```python
from build123d import *

# Parameters (mm, degrees)
CYLINDER023_R       = 1.8
CYLINDER023_DEPTH   = 20
ARRAY001003_X_COUNT = 2
ARRAY001003_X_PITCH = 31
ARRAY001003_Y_COUNT = 2
ARRAY001003_Y_PITCH = 31
CYLINDER020_R       = 13
CYLINDER020_DEPTH   = 30
CYLINDER024_R       = 30
CYLINDER024_DEPTH   = 30
CYLINDER039_R       = 1.45
CYLINDER039_DEPTH   = 40
ARRAY001020_X_COUNT = 2
ARRAY001020_X_PITCH = 20
ARRAY001021_X_COUNT = 2
ARRAY001021_X_PITCH = 90
CYLINDER041_R       = 1
CYLINDER041_DEPTH   = 10
ARRAY001023_Y_COUNT = 2
ARRAY001023_Y_PITCH = 92
CYLINDER022_R       = 4.1
CYLINDER022_DEPTH   = 24
ARRAY001002_X_COUNT = 2
ARRAY001002_X_PITCH = 90
ARRAY001002_Y_COUNT = 2
ARRAY001002_Y_PITCH = 50
CYLINDER025_R       = 7
CYLINDER025_DEPTH   = 25
ARRAY001004_X_COUNT = 2
ARRAY001004_X_PITCH = 90
ARRAY001004_Y_COUNT = 2
ARRAY001004_Y_PITCH = 50
BOX020_W            = 30
BOX020_H            = 100
BOX020_DEPTH        = 10
BOX002_W            = 120
BOX002_H            = 84
BOX002_DEPTH        = 10


with BuildPart() as motor_attachment_hole_array:
    # Cylinder023 → Cylinder023 (new body)
    with BuildSketch(Plane(origin=(84.5, 24.5, 0), x_dir=(1, 0, 0), z_dir=(0, 0, 1))):
        Circle(CYLINDER023_R)
    extrude(amount=CYLINDER023_DEPTH)

    # Array001003 X: motor attachment hole array ×2


with BuildPart() as motor_attachment_hole_array_1:
    add(motor_attachment_hole_array.part)
    with Locations(*[(i * ARRAY001003_X_PITCH, 0, 0) for i in range(1, ARRAY001003_X_COUNT)]):
        add(motor_attachment_hole_array.part)

    # Array001003 Y: motor attachment hole array ×2


with BuildPart() as motor_attachment_hole_array_2:
    add(motor_attachment_hole_array_1.part)
    with Locations(*[(0, i * ARRAY001003_Y_PITCH, 0) for i in range(1, ARRAY001003_Y_COUNT)]):
        add(motor_attachment_hole_array_1.part)


with BuildPart() as motor_hole_set_fusion:
    # Cylinder020 → Cylinder020 (new body)
    with BuildSketch(Plane(origin=(100, 40, -5), x_dir=(1, 0, 0), z_dir=(0, 0, 1))):
        Circle(CYLINDER020_R)
    extrude(amount=CYLINDER020_DEPTH)

    # Fusion010: union motor attachment hole array
    add(motor_attachment_hole_array_2.part)


with BuildPart() as central_hole001:
    # Cylinder024 → Cylinder024 (new body)
    with BuildSketch(Plane(origin=(49, 40, 0), x_dir=(1, 0, 0), z_dir=(0, 0, 1))):
        Circle(CYLINDER024_R)
    extrude(amount=CYLINDER024_DEPTH)


with BuildPart() as side_connector_narrow_hole_array_array:
    # Cylinder039 → Cylinder039 (new body)
    with BuildSketch(Plane.XZ):
        Circle(CYLINDER039_R)
    extrude(amount=CYLINDER039_DEPTH)

    # Array001020 X: side connector narrow hole array array ×2


with BuildPart() as side_connector_narrow_hole_array_array_1:
    add(side_connector_narrow_hole_array_array.part)
    with Locations(*[(i * ARRAY001020_X_PITCH, 0, 0) for i in range(1, ARRAY001020_X_COUNT)]):
        add(side_connector_narrow_hole_array_array.part)


with BuildPart() as side_connector_narrow_hole_array_array_2:
    # Array001020 placement: moved
    add(side_connector_narrow_hole_array_array_1.part.moved(Location((5, 0, 5))))

    # Array001021 X: side connector narrow hole array array ×2


with BuildPart() as side_connector_narrow_hole_array_array_3:
    add(side_connector_narrow_hole_array_array_2.part)
    with Locations(*[(i * ARRAY001021_X_PITCH, 0, 0) for i in range(1, ARRAY001021_X_COUNT)]):
        add(side_connector_narrow_hole_array_array_2.part)


with BuildPart() as side_connector_narrow_hole_array_array_4:
    # Array001021 placement: moved
    add(side_connector_narrow_hole_array_array_3.part.moved(Location((0, 27, 0))))


with BuildPart() as body009:
    # Body009 base: copy of side connector narrow hole array array
    add(side_connector_narrow_hole_array_array_4.part)


with BuildPart() as body009_1:
    # Body009 placement: moved
    add(body009.part.moved(Location((0, 67, 0))))


with BuildPart() as body010:
    # Body010 base: copy of side connector narrow hole array array
    add(side_connector_narrow_hole_array_array_4.part)


with BuildPart() as pusher_hole_array001:
    # Cylinder041 → Cylinder041 (new body)
    with BuildSketch(Plane(origin=(105, 0, 0), x_dir=(1, 0, 0), z_dir=(0, 0, 1))):
        Circle(CYLINDER041_R)
    extrude(amount=CYLINDER041_DEPTH)

    # Array001023 Y: pusher hole array001 ×2


with BuildPart() as pusher_hole_array001_1:
    add(pusher_hole_array001.part)
    with Locations(*[(0, i * ARRAY001023_Y_PITCH, 0) for i in range(1, ARRAY001023_Y_COUNT)]):
        add(pusher_hole_array001.part)


with BuildPart() as pusher_hole_array001_2:
    # Array001023 placement: moved
    add(pusher_hole_array001_1.part.moved(Location((0, -6, 0))))


with BuildPart() as motor_side_hole_fusion:
    # Cylinder022 → Cylinder022 (new body)
    with BuildSketch(Plane(origin=(14, 14, -30), x_dir=(1, 0, 0), z_dir=(0, 0, 1))):
        Circle(CYLINDER022_R)
    extrude(amount=CYLINDER022_DEPTH)

    # Array001002 X: motor side hole fusion ×2


with BuildPart() as motor_side_hole_fusion_1:
    add(motor_side_hole_fusion.part)
    with Locations(*[(i * ARRAY001002_X_PITCH, 0, 0) for i in range(1, ARRAY001002_X_COUNT)]):
        add(motor_side_hole_fusion.part)

    # Array001002 Y: motor side hole fusion ×2


with BuildPart() as motor_side_hole_fusion_2:
    add(motor_side_hole_fusion_1.part)
    with Locations(*[(0, i * ARRAY001002_Y_PITCH, 0) for i in range(1, ARRAY001002_Y_COUNT)]):
        add(motor_side_hole_fusion_1.part)

    # Fusion009: union motor hole set fusion, central hole001, Body009, Body010, pusher hole array001
    add(motor_hole_set_fusion.part)
    add(central_hole001.part)
    add(body009_1.part)
    add(body010.part)
    add(pusher_hole_array001_2.part)


with BuildPart() as rod_spacer_array:
    # Cylinder025 → Cylinder025 (new body)
    with BuildSketch(Plane(origin=(14, 14, -15), x_dir=(1, 0, 0), z_dir=(0, 0, 1))):
        Circle(CYLINDER025_R)
    extrude(amount=CYLINDER025_DEPTH)

    # Array001004 X: rod spacer array ×2


with BuildPart() as rod_spacer_array_1:
    add(rod_spacer_array.part)
    with Locations(*[(i * ARRAY001004_X_PITCH, 0, 0) for i in range(1, ARRAY001004_X_COUNT)]):
        add(rod_spacer_array.part)

    # Array001004 Y: rod spacer array ×2


with BuildPart() as rod_spacer_array_2:
    add(rod_spacer_array_1.part)
    with Locations(*[(0, i * ARRAY001004_Y_PITCH, 0) for i in range(1, ARRAY001004_Y_COUNT)]):
        add(rod_spacer_array_1.part)


with BuildPart() as motor_side_cube_extension:
    # Box020 → Box020 (new body)
    with BuildSketch(Plane(origin=(90, -10, 0), x_dir=(1, 0, 0), z_dir=(0, 0, 1))):
        with Locations((15, 50)):
            Rectangle(BOX020_W, BOX020_H)
    extrude(amount=BOX020_DEPTH)


with BuildPart() as motor_side_cut:
    # Box002 → Box002 (new body)
    with BuildSketch(Plane(origin=(0, -2, 0), x_dir=(1, 0, 0), z_dir=(0, 0, 1))):
        with Locations((60, 42)):
            Rectangle(BOX002_W, BOX002_H)
    extrude(amount=BOX002_DEPTH)

    # Fusion011: union rod spacer array, motor side cube extension
    add(rod_spacer_array_2.part)
    add(motor_side_cube_extension.part)

    # Cut003: cut motor side hole fusion
    add(motor_side_hole_fusion_2.part, mode=Mode.SUBTRACT)


solid = motor_side_cut.part
```
Here's how the part is built. I have some questions about the finished solid (model axes, mm). A direction names the side the tool comes from. Coordinates: 2 decimals unless noted, no trailing zeros. Write each loop counter-clockwise with the first axis right and the second up, starting at its lowest first coordinate (ties: lowest second). Pieces come first, ordered by that corner, then holes. Notation, with made-up numbers: (68, 57.5) -> (95, 57.5) arc R29 cw to (95, 77.5) -> close; hole circle Ø10 at (83.25, -33.75). An arc over 180 degrees is marked (long way). Use a Markdown table: item, result. Add a question column.
(1) I'm going to push flat-ended pins straight in: P1, Ø2.5, axis at x = 115, z = 5, coming from the -Y side; P2, Ø3, axis at x = 84.5, y = 24.5, coming from the -Z side; P3, Ø11, axis at x = 29.5, z = 5, coming from the +Y side; P4, Ø4, axis at x = 14, y = 14.5, coming from the -Z side. Where does each tip first touch, or does it pass through?
(2) If we section it at C-C, the plane x = 95: Write out the boundary of the cut face in (y, z), and give its area (3 significant figures).
(3) We'd pull the mould along Z, two halves only. Please class faces 1 (the flat face through (95, 54, 5)), 2 (the flat face through (104, 64, -6)), 3 (the flat face through (44, 82, 5)): +Z half, -Z half, draft (parallel to the pull), parting line (faces both ways), or undercut.
(4) If we section it at D-D, the plane y = 40: Write out the boundary of the cut face in (x, z), and give its area (3 significant figures).
(5) If we section it at A-A, the plane z = -9: Write out the boundary of the cut face in (x, y), and give its area (3 significant figures).
(6) Please list where these lines run through material, in increasing order: line 1 (X direction, y = 64, z = -9.5); line 2 (X direction, y = 75.5, z = 5); line 3 (X direction, y = 39.5, z = 7.75).
(7) For faces 4 (the cylindrical face through (13.09, 70.94, -7.6)), 5 (the flat face through (95, 27, 5)), 6 (the flat face through (44, -2, 5)), which set-ups out of +Z, -Z, +X, -X, +Y, -Y let a thin tool reach every point of the face, with its end or its side?
(8) If we section it at B-B, the plane y = 64: Write out the boundary of the cut face in (x, z), and give its area (3 significant figures).
Outcome:
| question | item | result |
|---|---|---|
| 1 | P1 | stops at y = 27 |
| 1 | P2 | passes through |
| 1 | P3 | stops at y = 82 |
| 1 | P4 | stops at z = -6 |
| 2 | outline | (-10, 0) -> (28, 0) -> (28, 10) -> (-10, 10) -> (-10, 6.45) -> (27, 6.45) -> (27, 3.55) -> (-10, 3.55) -> close; (52, 0) -> (90, 0) -> (90, 3.55) -> (54, 3.55) -> (54, 6.45) -> (90, 6.45) -> (90, 10) -> (52, 10) -> close |
| 2 | area | 548 mm^2 |
| 3 | face 1 | undercut |
| 3 | face 2 | -Z half |
| 3 | face 3 | draft |
| 4 | outline | (0, 0) -> (19, 0) -> (19, 10) -> (0, 10) -> close; (79, 0) -> (87, 0) -> (87, 10) -> (79, 10) -> close; (113, 0) -> (120, 0) -> (120, 10) -> (113, 10) -> close |
| 4 | area | 340 mm^2 |
| 5 | outline | circle Ø14 at (14, 14); circle Ø14 at (14, 64); circle Ø14 at (104, 14); circle Ø14 at (104, 64); hole circle Ø8.2 at (14, 14); hole circle Ø8.2 at (14, 64); hole circle Ø8.2 at (104, 14); hole circle Ø8.2 at (104, 64) |
| 5 | area | 405 mm^2 |
| 6 | line 1 | x = 7 to 9.9, 18.1 to 21, 97 to 99.9, 108.1 to 111 |
| 6 | line 2 | x = 0 to 3.55, 6.45 to 23.55, 26.45 to 93.55, 96.45 to 113.55, 116.45 to 120 |
| 6 | line 3 | x = 0 to 19, 79 to 87.01, 112.99 to 120 |
| 7 | face 4 | -Z |
| 7 | face 5 | -Y |
| 7 | face 6 | +Z, -Z, -X, -Y |
| 8 | outline | (0, 0) -> (7, 0) -> (7, -15) -> (9.9, -15) -> (9.9, -6) -> (18.1, -6) -> (18.1, -15) -> (21, -15) -> (21, 0) -> (31, 0) -> (31, 10) -> (0, 10) -> close; (67, 0) -> (97, 0) -> (97, -15) -> (99.9, -15) -> (99.9, -6) -> (108.1, -6) -> (108.1, -15) -> (111, -15) -> (111, 0) -> (120, 0) -> (120, 10) -> (67, 10) -> close; hole circle Ø2.9 at (5, 5); hole circle Ø2.9 at (25, 5); hole circle Ø2.9 at (95, 5); hole circle Ø2.9 at (115, 5) |
| 8 | area | 1,090 mm^2 |
